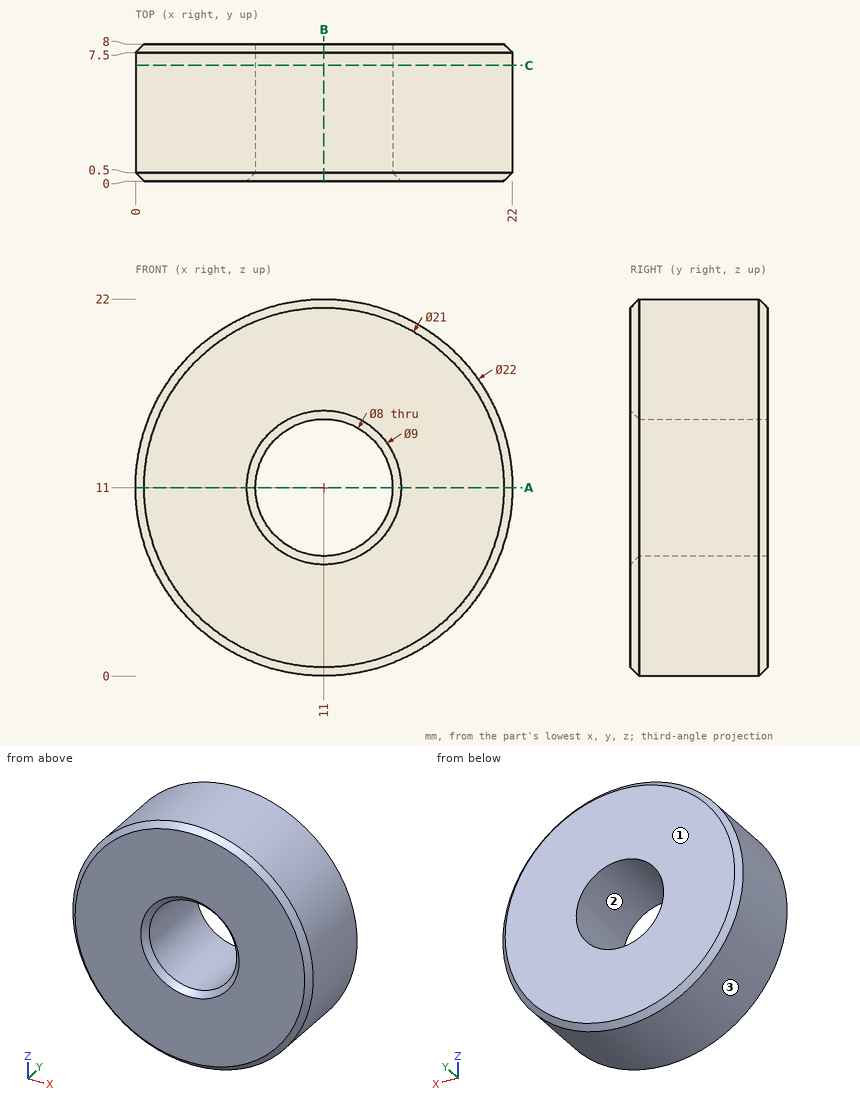
Study the drawing (mm; zero at the part's minimum x, y, z) and answer. Give positions to 0.01 mm unless a question says otherwise; leave off trailing zeros. Write each loop counter-clockwise with the first axis right and the second up, starting at its lowest first coordinate (ties: lowest second). Pieces come first, ordered by that corner, then holes. Notation, with made-up numbers: (41.25, 81) -> (100.25, 81) arc R29 cw to (100.25, 116) -> close; hole circle Ø7 at (87, 1). An arc over 180 degrees is marked (long way). Write item = value, one per line. Start each with the question number.
1) The part is cut by section B-B, the plane x = 11. Determine the outline of the cut face in (y, z), and give its area (3 significant figures).
2) Determine the mould class of the marked faces 1, 2 and 3 for opening direction Z: +Z half, -Z half, draft (parallel to the pull), parting line (faces both ways), or undercut.
3) Each of these flat-tipped pins is pushed along its axis until it touches: pin 1 (5 mm diameter, centred on x = 11, z = 11, fed in from +Y); pin 2 (2 mm diameter, centred on x = 4.5, y = 6.5, fed in from +Z). Where does it stop, or does it pass through?
4) Straight lines are drawn through the part: line 1 along X through (y, z) = (4.5, 11); line 2 along X through (y, z) = (2.75, 14); line 3 along Z through (x, y) = (8.75, 1). For each, find the intervals that lie inside material, in ascending order.
5) The part is cut by section A-A, the plane z = 11. Determine the outline of the cut face in (x, y), and give its area (3 significant figures).
6) The part is cut by section C-C, the plane y = 6.75. Determine the outline of the cut face in (x, z), and give its area (3 significant figures).
Solutions:
q1.outline = (0, 0.5) -> (0.5, 0) -> (7.5, 0) -> (8, 0.5) -> (8, 7) -> (0.5, 7) -> (0, 6.5) -> close; (0, 15.5) -> (0.5, 15) -> (8, 15) -> (8, 21.5) -> (7.5, 22) -> (0.5, 22) -> (0, 21.5) -> close
q1.area = 111 mm²
q2.face_1 = draft
q2.face_2 = undercut
q2.face_3 = parting line
q3.pin_1 = through
q3.pin_2 = 20.53
q4.line_1 = 0 to 7, 15 to 22
q4.line_2 = 0.42 to 8.35, 13.65 to 21.58
q4.line_3 = 0.23 to 7.69, 14.31 to 21.77
q5.outline = (0, 0.5) -> (0.5, 0) -> (6.5, 0) -> (7, 0.5) -> (7, 8) -> (0.5, 8) -> (0, 7.5) -> close; (15, 0.5) -> (15.5, 0) -> (21.5, 0) -> (22, 0.5) -> (22, 7.5) -> (21.5, 8) -> (15, 8) -> close
q5.area = 111 mm²
q6.outline = circle Ø22 at (11, 11); hole circle Ø8 at (11, 11)
q6.area = 330 mm²
